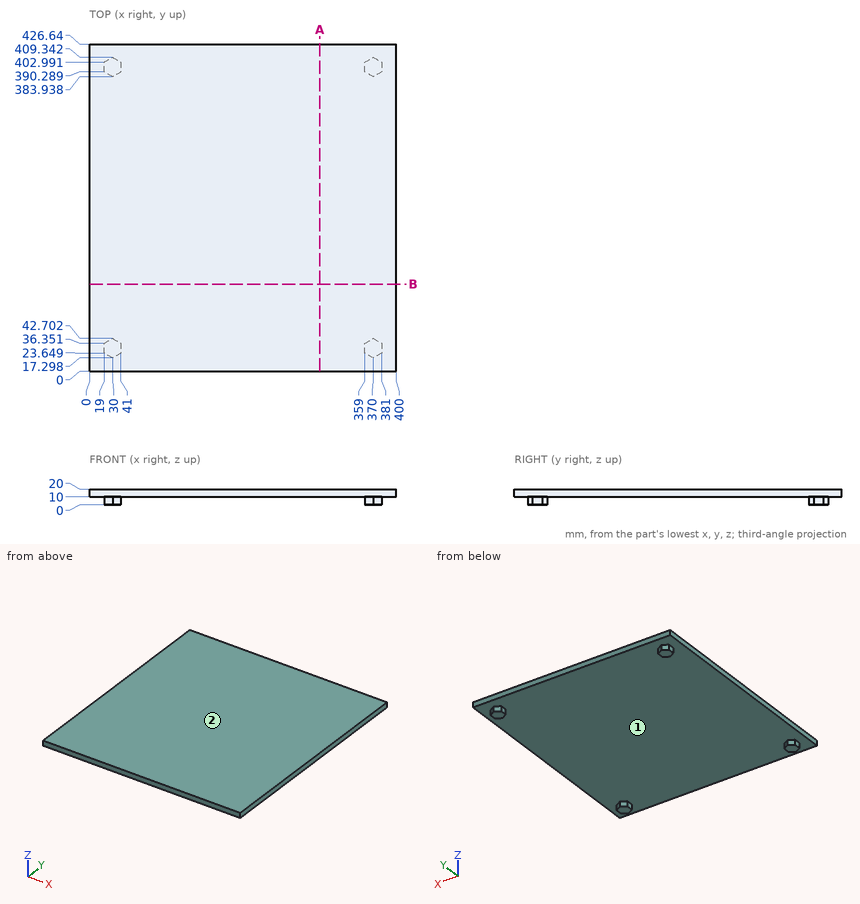
Print and shaded views of the part. All mm, measured from the part's lowest x, y and z. Round coordinates to 2 decimals unless told otherwise and drop trailing zeros. Write each loop counter-clockwise with the first axis right and the second up, starting at its lowest first coordinate (ties: lowest second). Pieces come first, ordered by that corner, then holes. Notation, with made-up numbers: (26, -39) -> (49, -39) arc R20 ccw to (49, -14) -> close; hole circle Ø2 at (-15.75, 58.5). An arc over 180 degrees is marked (long way). Answer in a Markdown table with one row per item. Add a question column.
Item 1: Drop flat-ended pins along their axis: pin 1 Ø11 at (y, z) = (397, 4) entering from -X; pin 2 Ø10 at (x, y) = (158, 314) entering from -Z; pin 3 Ø4 at (x, z) = (333, 13.5) entering from -Y; pin 4 Ø5 at (y, z) = (399, 6) entering from +X. Give the stop position or say it passes through.
Item 2: Saw through at A-A, the plane x = 300.5. Write the cut outline in (y, z), then the cut area to 3 significant figures.
Item 3: Saw through at B-B, the plane y = 113.5. Write the cut outline in (x, z).
Item 4: Drill centre lines: line 1 (Z direction, x = 359.5, y = 213.5); line 2 (X direction, y = 22, z = 6.5) (1 decimal); line 3 (X direction, y = 406, z = 2.75). Where is each one in solid material? Low to high. Write a range as from..to.
Item 5: Mould opens along X. For the marked faces 1 and 2 say: pulls with the +X half, pulls with the -X half, needs draft (parallel to the pull), parting line crosses it, or undercut.
Findings below:
| question | item | result |
|---|---|---|
| 1 | pin 1 | stops at x = 19 |
| 1 | pin 2 | stops at z = 10 |
| 1 | pin 3 | stops at y = 0 |
| 1 | pin 4 | stops at x = 381 |
| 2 | outline | (0, 10) -> (426.64, 10) -> (426.64, 20) -> (0, 20) -> close |
| 2 | area | 4,270 mm^2 |
| 3 | outline | (0, 10) -> (400, 10) -> (400, 20) -> (0, 20) -> close |
| 4 | line 1 | z = 10..20 |
| 4 | line 2 | x = 21.9..38.1, 361.9..378.1 |
| 4 | line 3 | x = 24.21..35.79, 364.21..375.79 |
| 5 | face 1 | undercut |
| 5 | face 2 | needs draft |
